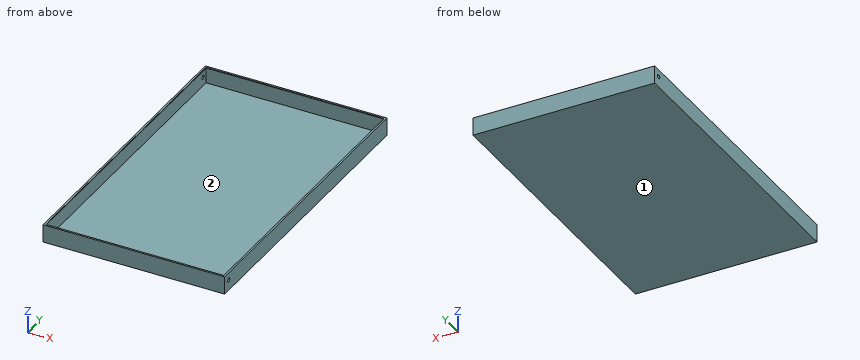
```python
from build123d import *

# Parameters (mm, degrees)
SKETCH1_W           = 1000
SKETCH1_H           = 1662.9
BOSS_EXTRUDE1_DEPTH = 10
SKETCH2_W           = 1020
SKETCH2_H           = 1682.9
SKETCH2_W_2         = 1000
SKETCH2_H_2         = 1662.9
BOSS_EXTRUDE2_DEPTH = 100
CUT_EXTRUDE1_REACH  = 1963.885
SKETCH3_R           = 11.45
SKETCH4_R           = 11.45
CUT_EXTRUDE2_DEPTH  = 10
SKETCH6_W           = 1000
SKETCH6_H           = 1662.9
SKETCH6_W_2         = 996
SKETCH6_H_2         = 1658.9
BOSS_EXTRUDE4_DEPTH = 2


with BuildPart() as part:
    # Sketch1 → Boss-Extrude1 (new body)
    with BuildSketch(Plane.XY):
        with Locations((500, 831.45)):
            Rectangle(SKETCH1_W, SKETCH1_H)
    extrude(amount=BOSS_EXTRUDE1_DEPTH)

    # Sketch2 → Boss-Extrude2 (add)
    with BuildSketch(Plane.XY):
        with Locations((500, 831.45)):
            Rectangle(SKETCH2_W, SKETCH2_H)
        with Locations((500, 831.45)):
            Rectangle(SKETCH2_W_2, SKETCH2_H_2, mode=Mode.SUBTRACT)
    extrude(amount=BOSS_EXTRUDE2_DEPTH)

    # Sketch3 → Cut-Extrude1 (cut, up to next)
    with BuildSketch(Plane.ZY.offset(10), mode=Mode.PRIVATE) as cut_extrude1_sk1:
        with Locations(Location((60, 1631.45, 0), (0, 0, 270))):
            Circle(SKETCH3_R)
    cut_extrude1_tool1 = extrude(cut_extrude1_sk1.sketch, amount=-CUT_EXTRUDE1_REACH, mode=Mode.PRIVATE) & part.part
    add(cut_extrude1_tool1.solids().sort_by_distance((-10, 1631.45, 60))[0], mode=Mode.SUBTRACT)

    # Sketch4 → Cut-Extrude2 (cut)
    with BuildSketch(Plane(origin=(1010, 0, 0), x_dir=(0, 0, -1), z_dir=(1, 0, 0))):
        with Locations(Location((-60, 31.47, 0), (0, 0, 90))):
            Circle(SKETCH4_R)
    extrude(amount=-CUT_EXTRUDE2_DEPTH, mode=Mode.SUBTRACT)

    # Sketch6 → Boss-Extrude4 (add)
    with BuildSketch(Plane.XY.offset(98)):
        with Locations((500, 831.45)):
            Rectangle(SKETCH6_W, SKETCH6_H)
        with Locations((500, 831.45)):
            Rectangle(SKETCH6_W_2, SKETCH6_H_2, mode=Mode.SUBTRACT)
    extrude(amount=-BOSS_EXTRUDE4_DEPTH)


solid = part.part
```
Model file for the job. Use its own axes, mm. Face numbers are marked on the shaded views. Round coordinates to 2 decimals unless told otherwise and drop trailing zeros. Order: outer loops, then holes, each group sorted by start corner. A loop starts at its lowest first (then second) coordinate and runs counter-clockwise, first axis right, second up. Notation, with made-up numbers: (46, 76) -> (74, 76) arc R11 cw to (74, 85) -> close; hole circle Ø9 at (76.25, 18.5). An arc over 180 degrees is marked (long way). Use one line per item in the form item = value.
Item 1: Cut at B-B, the plane y = 1540.5. Write the cut outline in (x, z), and give its area (3 significant figures).
Returned:
outline = (-10, 0) -> (1010, 0) -> (1010, 100) -> (1000, 100) -> (1000, 98) -> (998, 98) -> (998, 96) -> (1000, 96) -> (1000, 10) -> (0, 10) -> (0, 96) -> (2, 96) -> (2, 98) -> (0, 98) -> (0, 100) -> (-10, 100) -> close
area = 12,000 mm^2
Item 2: Drill centre lines: line 1 (Z direction, x = 1007.25, y = 31.47); line 2 (Y direction, x = 237, z = 68); line 3 (X direction, y = 193, z = 26). Where is each one in solid material? Low to high.
Returned:
line_1 = 0 to 48.55, 71.45 to 100
line_2 = -10 to 0, 1662.9 to 1672.9
line_3 = -10 to 0, 1000 to 1010
Item 3: Pull direction X, two halves, no side cores. Call the marked faces 1 and 2: released by +X, released by -X, zero draft, split by the parting line, or undercut.
Returned:
face_1 = zero draft
face_2 = undercut
Item 4: Cut at C-C, the plane x = 941. Write the cut outline in (y, z).
Returned:
outline = (-10, 0) -> (1672.9, 0) -> (1672.9, 100) -> (1662.9, 100) -> (1662.9, 98) -> (1660.9, 98) -> (1660.9, 96) -> (1662.9, 96) -> (1662.9, 10) -> (0, 10) -> (0, 96) -> (2, 96) -> (2, 98) -> (0, 98) -> (0, 100) -> (-10, 100) -> close
Item 5: Cut at A-A, the plane z = 25.5. Write the cut outline in (x, y), and give its area (3 significant figures).
Returned:
outline = (-10, -10) -> (1010, -10) -> (1010, 1672.9) -> (-10, 1672.9) -> close; hole (0, 0) -> (1000, 0) -> (1000, 1662.9) -> (0, 1662.9) -> close
area = 53,700 mm^2
Item 6: Flat gauge pins, fed straight in: pin 1 Ø3 at (x, y) = (103.5, 1176.5) entering from +Z; pin 2 Ø20.5 at (y, z) = (31.47, 60) entering from +X; pin 3 Ø12 at (x, y) = (241, 379) entering from -Z. Where does each tip first touch, or does it go through?
Returned:
pin_1 = 10
pin_2 = 0
pin_3 = 0
